from build123d import *

# Parameters (mm, degrees)
SKETCH1_R           = 53
SKETCH1_R_2         = 43
BOSS_EXTRUDE1_DEPTH = 20
SKETCH2_R           = 43
BOSS_EXTRUDE2_DEPTH = 20
SKETCH3_R           = 47.5
CUT_EXTRUDE1_DEPTH  = 8
SKETCH4_R           = 47.5
CUT_EXTRUDE2_DEPTH  = 8
SKETCH5_R           = 3
SKETCH5_R_2         = 5
CUT_EXTRUDE3_DEPTH  = 13


with BuildPart() as part:
    # Sketch1 → Boss-Extrude1 (new body)
    with BuildSketch(Plane(origin=(0, 0, 0), x_dir=(1, 0, 0), z_dir=(0, 1, 0))):
        Circle(SKETCH1_R)
        Circle(SKETCH1_R_2, mode=Mode.SUBTRACT)
    extrude(amount=BOSS_EXTRUDE1_DEPTH)

    # Sketch2 → Boss-Extrude2 (add)
    with BuildSketch(Plane(origin=(0, 20, 0), x_dir=(1, 0, 0), z_dir=(0, 1, 0))):
        Circle(SKETCH2_R)
    extrude(amount=-BOSS_EXTRUDE2_DEPTH)

    # Sketch3 → Cut-Extrude1 (cut)
    with BuildSketch(Plane(origin=(0, 20, 0), x_dir=(1, 0, 0), z_dir=(0, 1, 0))):
        Circle(SKETCH3_R)
    extrude(amount=-CUT_EXTRUDE1_DEPTH, mode=Mode.SUBTRACT)

    # Sketch4 → Cut-Extrude2 (cut)
    with BuildSketch(Plane.XZ):
        Circle(SKETCH4_R)
    extrude(amount=-CUT_EXTRUDE2_DEPTH, mode=Mode.SUBTRACT)

    # Sketch5 → Cut-Extrude3 (cut, through all)
    with BuildSketch(Plane(origin=(0, 12, 0), x_dir=(1, 0, 0), z_dir=(0, 1, 0))):
        Circle(SKETCH5_R)
        with Locations((0, 35)):
            Circle(SKETCH5_R_2)
        with Locations((24.748737342, 24.748737342)):
            Circle(SKETCH5_R_2)
        with Locations((35, 0)):
            Circle(SKETCH5_R_2)
        with Locations((24.748737342, -24.748737342)):
            Circle(SKETCH5_R_2)
        with Locations((0, -35)):
            Circle(SKETCH5_R_2)
        with Locations((-24.748737342, -24.748737342)):
            Circle(SKETCH5_R_2)
        with Locations((-35, 0)):
            Circle(SKETCH5_R_2)
        with Locations((-24.748737342, 24.748737342)):
            Circle(SKETCH5_R_2)
    extrude(amount=-CUT_EXTRUDE3_DEPTH, mode=Mode.SUBTRACT)


solid = part.part
Design review of the part built by this model. Coordinates are the model's own, in mm. A direction names the side the tool comes from. Round coordinates to 2 decimals unless told otherwise and drop trailing zeros. Write each loop counter-clockwise with the first axis right and the second up, starting at its lowest first coordinate (ties: lowest second). Pieces come first, ordered by that corner, then holes. Notation, with made-up numbers: (15.5, -34) - (51.5, -34) arc R4 ccw to (51.5, -28) - close; hole circle Ø6 at (54, 25). An arc over 180 degrees is marked (long way). Return JSON: item names as keys, results as strings. Group by question number.
Item 1: We need section A-A on z = 0. Write out the cut boundary in (x, y).
Item 2: The part is to be moulded in two halves that separate along Z. For faces 1 (the face through (28, 10, -45)), 2 (the face through (-43.4, 20, -19.9)), 3 (the face through (10, 12, -1)), say which applies: pulls with the +Z half, pulls with the -Z half, needs draft (parallel to the pull), parting line crosses it, or undercut.
Item 3: For probe 1 along Z at (x, y) = (0, 16); probe 2 along Z at (x, y) = (27.5, 8.25); probe 3 along Y at (x, z) = (20, 9), list the stretches that pass through material, from the lowest coordinate up. Write a range as [from, to].
Item 4: We need section B-B on x = 0. Write out the cut boundary in (y, z), and give its area (3 significant figures).
Item 5: Insertion check: P1, Ø5, axis at x = 28.5, z = 4.5, coming from the -Y side; P2, Ø9.5, axis at x = 0, z = 0, coming from the +Y side; P3, Ø3, axis at y = 11.5, z = 18.5, coming from the -X side; P4, Ø12, axis at x = 42.5, z = -38.5, coming from the +Y side. Each pin has a flat end and moves straight along its axis. Give the tip position at first contact, or say it passes through.
Item 6: We need section D-D on x = -35. Write out the cut boundary in (y, z).
Item 7: Machinability: for faces 4 (the face through (10, 8, 1)), 5 (the face through (-10.3, 16.06, 46.37)), 6 (the face through (-43.4, 0, -19.9)), which of the approach directions +Z, -Z, +X, -X, +Y, -Y give a long, thin tool a straight path to every point of the face, cutting with its end or side? Answer none if there is none.
Item 8: We need section C-C on z = 26. Write out the cut boundary in (x, y), and give its area (3 significant figures).
Model answer:
{
 "1": {"outline": "(-53, 0) - (-47.5, 0) - (-47.5, 8) - (-40, 8) - (-40, 12) - (-47.5, 12) - (-47.5, 20) - (-53, 20) - close; (-30, 8) - (-3, 8) - (-3, 12) - (-30, 12) - close; (3, 8) - (30, 8) - (30, 12) - (3, 12) - close; (40, 8) - (47.5, 8) - (47.5, 0) - (53, 0) - (53, 20) - (47.5, 20) - (47.5, 12) - (40, 12) - close"},
 "2": {"face 1": "parting line crosses it", "face 2": "needs draft", "face 3": "undercut"},
 "3": {"probe 1": "z = [-53, -47.5], [47.5, 53]", "probe 2": "z = [-45.31, -28.92], [-20.57, 20.57], [28.92, 45.31]", "probe 3": "y = [8, 12]"},
 "4": {"outline": "(0, -53) - (20, -53) - (20, -47.5) - (12, -47.5) - (12, -40) - (8, -40) - (8, -47.5) - (0, -47.5) - close; (0, 47.5) - (8, 47.5) - (8, 40) - (12, 40) - (12, 47.5) - (20, 47.5) - (20, 53) - (0, 53) - close; (8, -30) - (12, -30) - (12, -3) - (8, -3) - close; (8, 3) - (12, 3) - (12, 30) - (8, 30) - close", "area": "496 mm²"},
 "5": {"P1": "stops at y = 8", "P2": "stops at y = 12", "P3": "stops at x = -50.2", "P4": "stops at y = 20"},
 "6": {"outline": "(0, -39.8) - (20, -39.8) - (20, -32.11) - (12, -32.11) - (12, -5) - (8, -5) - (8, -32.11) - (0, -32.11) - close; (0, 32.11) - (8, 32.11) - (8, 5) - (12, 5) - (12, 32.11) - (20, 32.11) - (20, 39.8) - (0, 39.8) - close"},
 "7": {"face 4": "-Y", "face 5": "+Y", "face 6": "+Z, -Z, +X, -X, -Y"},
 "8": {"outline": "(-46.18, 0) - (-39.75, 0) - (-39.75, 8) - (-29.59, 8) - (-29.59, 12) - (-39.75, 12) - (-39.75, 20) - (-46.18, 20) - close; (-19.91, 8) - (19.91, 8) - (19.91, 12) - (-19.91, 12) - close; (29.59, 8) - (39.75, 8) - (39.75, 0) - (46.18, 0) - (46.18, 20) - (39.75, 20) - (39.75, 12) - (29.59, 12) - close", "area": "498 mm²"}
}
